Part model, mm, in its own coordinate system. Face numbers are marked on the shaded views. Give positions to 0.01 mm unless a question says otherwise; leave off trailing zeros. Order: outer loops, then holes, each group sorted by start corner. A loop starts at its lowest first (then second) coordinate and runs counter-clockwise, first axis right, second up. Notation, with made-up numbers: M 69,38.25 L 91,38.25 A21 cw 91,76.25 Z; hole C 5,84 d2. An arc over 180 degrees is marked long. One line per question, with ' | ' between items.
```python
from build123d import *

# Parameters (mm, degrees)
SKETCH1_R           = 15.875
SKETCH1_R_2         = 2.1828125
SKETCH1_W           = 3.175
SKETCH1_H           = 3.175
BOSS_EXTRUDE1_DEPTH = 12.7


with BuildPart() as part:
    # Sketch1 → Boss-Extrude1 (new body)
    with BuildSketch(Plane(origin=(0, 0, 0), x_dir=(1, 0, 0), z_dir=(0, 1, 0))):
        with Locations(Location((0, 0, 0), (0, 0, 270))):
            Circle(SKETCH1_R)
        with Locations(Location((12.7, 0, 0), (0, 0, 270))):
            Circle(SKETCH1_R_2, mode=Mode.SUBTRACT)
        with Locations(Location((-12.7, 0, 0), (0, 0, 270))):
            Circle(SKETCH1_R_2, mode=Mode.SUBTRACT)
        Rectangle(SKETCH1_W, SKETCH1_H, mode=Mode.SUBTRACT)
    extrude(amount=BOSS_EXTRUDE1_DEPTH)


solid = part.part
```
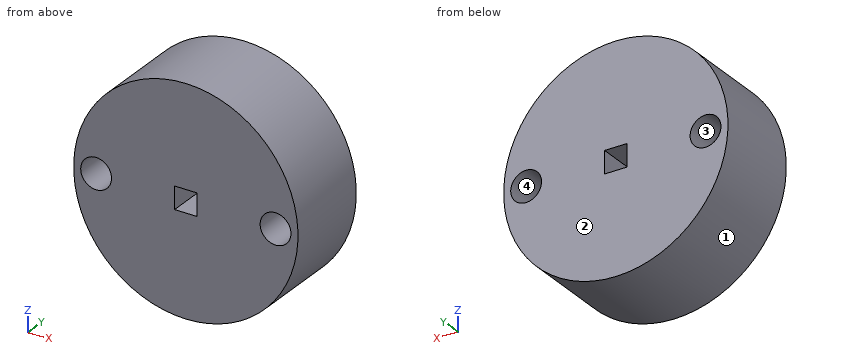
1. Mould opens along Z. For the marked faces 1, 2, 3 and 4 say: released by +Z, released by -Z, zero draft, split by the parting line, or undercut.
Worked out:
face 1: split by the parting line | face 2: zero draft | face 3: undercut | face 4: undercut
2. Slice it at C-C on x = 0. Give the cut face in (y, z) (1 decimal), then the cut area to 3 significant figures.
Worked out:
outline: M 0,-15.9 L 12.7,-15.9 L 12.7,-1.6 L 0,-1.6 Z; M 0,1.6 L 12.7,1.6 L 12.7,15.9 L 0,15.9 Z | area: 363 mm2
3. Slice it at B-B on z = 0. Give the cut face in (x, y) (1 decimal).
Worked out:
outline: M -15.9,0 L -14.9,0 L -14.9,12.7 L -15.9,12.7 Z; M -10.5,0 L -1.6,0 L -1.6,12.7 L -10.5,12.7 Z; M 1.6,0 L 10.5,0 L 10.5,12.7 L 1.6,12.7 Z; M 14.9,0 L 15.9,0 L 15.9,12.7 L 14.9,12.7 Z
4. Drop flat-ended pins along their axis: pin 1 (1.5 mm diameter, centred on y = 8, z = -9.5, fed in from +X); pin 2 (5 mm diameter, centred on x = 5.5, y = 11, fed in from -Z); pin 3 (1.5 mm diameter, centred on x = -4.5, y = 5.5, fed in from -Z). Give the stop position or say it passes through.
Worked out:
pin 1: stops at x = 13.25 | pin 2: stops at z = -15.59 | pin 3: stops at z = -15.43
5. Slice it at D-D on x = -12.7. Give the cut face in (y, z) (3 decimals).
Worked out:
outline: M 0,-9.525 L 12.7,-9.525 L 12.7,-2.183 L 0,-2.183 Z; M 0,2.183 L 12.7,2.183 L 12.7,9.525 L 0,9.525 Z
6. Probe L1, parallel to X at y = 3.25, z = 0 (1 decimal); L2, parallel to X at y = 6, z = -1; L3, parallel to X at y = 10.5, z = -2. List the from-to ranges inside material, lowest first. Write a range as from..to.
Worked out:
L1: x = -15.9..-14.9, -10.5..-1.6, 1.6..10.5, 14.9..15.9 | L2: x = -15.84..-14.64, -10.76..-1.59, 1.59..10.76, 14.64..15.84 | L3: x = -15.75..-13.57, -11.83..11.83, 13.57..15.75
7. Slice it at A-A on y = 6.75. Give the number of separate pieces and of enclosed holes in the cut face, then the cut area to 3 significant figures.
Worked out:
separate pieces: 1 | enclosed holes: 3 | area: 752 mm2
